```python
from build123d import *

# Parameters (mm, degrees)
EXTRUDE_1_DEPTH              = 7
CUT_EXTRUDE_1_DEPTH          = 4
HOLE_WIZARD_M3_1_D           = 3.4
HOLE_WIZARD_M3_1_DEPTH       = 7.5
HOLE_WIZARD_M3_1_CSINK_D     = 6.72
HOLE_WIZARD_M3_1_CSINK_ANGLE = 90
HOLE_WIZARD_M3_1_TIP         = 1.021463052
HOLE_WIZARD_1_D              = 4.15
CUT_EXTRUDE_2_DEPTH          = 4
CHAMFER_1_SIZE               = 0.5


with BuildPart() as part:
    # 草图1 → 凸台-拉伸1 (new body)
    with BuildSketch(Plane(origin=(0, 0, 0), x_dir=(1, 0, 0), z_dir=(0, 1, 0))):
        with BuildLine():
            Line((-4.25, 5), (4.25, 5))
            ThreePointArc((4.25, 5), (9.25, 0), (4.25, -5))
            Line((4.25, -5), (-4.25, -5))
            ThreePointArc((-4.25, -5), (-9.25, 0), (-4.25, 5))
        make_face()
    extrude(amount=EXTRUDE_1_DEPTH)

    # 草图2 → 切除-拉伸1 (cut)
    with BuildSketch(Plane(origin=(0, 7, 0), x_dir=(1, 0, 0), z_dir=(0, 1, 0))):
        with BuildLine():
            Line((-2.75, 2), (-5.75, 2))
            ThreePointArc((-5.75, 2), (-6.75, 0), (-5.75, -2))
            Line((-5.75, -2), (-2.75, -2))
            ThreePointArc((-2.75, -2), (-2.013932023, -1.118033989), (-1.75, 0))
            ThreePointArc((-1.75, 0), (-2.013932023, 1.118033989), (-2.75, 2))
        make_face()
    extrude(amount=-CUT_EXTRUDE_1_DEPTH, mode=Mode.SUBTRACT)

    # M3 六角凹锥坑螺钉的锥形沉头孔1
    with Locations(Plane(origin=(0, 0, 0), x_dir=(-1, 0, 0), z_dir=(0, -1, 0))):
        with Locations((4.25, 0)):
            CounterSinkHole(HOLE_WIZARD_M3_1_D / 2, HOLE_WIZARD_M3_1_CSINK_D / 2, depth=HOLE_WIZARD_M3_1_DEPTH, counter_sink_angle=HOLE_WIZARD_M3_1_CSINK_ANGLE)
            with Locations((0, 0, -(HOLE_WIZARD_M3_1_DEPTH + HOLE_WIZARD_M3_1_TIP / 2))):  # 118° drill point
                Cone(0, HOLE_WIZARD_M3_1_D / 2, HOLE_WIZARD_M3_1_TIP, mode=Mode.SUBTRACT)

    # 孔1 (through all)
    with Locations(Plane(origin=(0, 7, 0), x_dir=(1, 0, 0), z_dir=(0, 1, 0))):
        with Locations((5, -0.436816998)):
            Hole(HOLE_WIZARD_1_D / 2)

    # 草图12 → 切除-拉伸2 (cut)
    with BuildSketch(Plane(origin=(0, 7, 0), x_dir=(1, 0, 0), z_dir=(0, 1, 0))):
        Polygon((8.348631561, -0.436816998), (6.674315781, 2.463183002), (3.325684219, 2.463183002), (1.651368439, -0.436816998), (3.325684219, -3.336816998), (6.674315781, -3.336816998), align=None)
    extrude(amount=-CUT_EXTRUDE_2_DEPTH, mode=Mode.SUBTRACT)

    # 倒角1
    chamfer_1_edges = [part.edges().sort_by_distance(p)[0] for p in [
        (9.25, 7, 0),
        (0, 7, -5),
        (-9.25, 7, 0),
        (0, 0, -5),
        (9.25, 0, 0),
        (0, 0, 5),
        (-9.25, 0, 0),
        (0, 7, 5),
    ]]
    chamfer(chamfer_1_edges, length=CHAMFER_1_SIZE)


solid = part.part
```
Source: CAD feature listing. Evaluate the final solid. Frame: model axes, mm. A direction names the side the tool comes from. Round coordinates to 2 decimals unless told otherwise and drop trailing zeros. Loops run counter-clockwise (first coordinate to the right, second up) from the corner with the lowest first, then second, coordinate; pieces in that order, holes last. Notation, with made-up numbers: M 20.25,53 L 26.25,53 A19 cw 26.25,57 Z; hole C -24.75,78.5 d9. An arc over 180 degrees is marked long. Use a Markdown table: item, result. Add a question column.
1. Contact query for flat-ended pins moving along their axis: P1, Ø5, axis at x = 4.5, z = -2, coming from the +Y side; P2, Ø1.2, axis at x = -3, z = 0.5, coming from the +Y side; P3, Ø4, axis at x = -4.25, z = 0, coming from the -Y side; P4, Ø1, axis at x = 4, z = 0.5, coming from the +Y side. Output: stop coordinate, or through.
2. Reachability of faces 4 (the flat face through (5, 5, -2.463)), 5 (the cylindrical face through (-9.25, 3.46, 0.11)) from +Z, -Z, +X, -X, +Y, -Y: full face, straight path, thin tool, end or side. Return the list, or none.
3. Section query D-D on z = -1. Give the number of separate pieces and of enclosed holes in the cut face, then the cut area to 3 significant figures.
4. Mould query, pull axis X, two halves, no side actions, for faces 1 (the cylindrical face through (9.25, 3.46, -0.11)), 2 (the flat face through (5, 5, 3.337)), 3 (the conical face through (-8.884, 6.865, 0.102)). Classes: pulls with the +X half, pulls with the -X half, needs draft (parallel to the pull), parting line crosses it, or undercut.
5. Section query A-A on y = 5.75. Return the cut outline in (x, z), then the cut area to 3 significant figures.
6. Section query C-C on y = 2. Return the cut outline in (x, z) (3 decimals), then the cut area to 3 significant figures.
7. Line query: line 1 (X direction, y = 2.75, z = 1.25); line 2 (X direction, y = 4.5, z = -0.25); line 3 (Z direction, x = -3.25, y = 4.25). Output: solid intervals per line, ascending.
8. Section query B-B on x = 4. Return the cut outline in (y, z).
Reported:
| question | item | result |
|---|---|---|
| 1 | P1 | stops at y = 7 |
| 1 | P2 | stops at y = 3 |
| 1 | P3 | stops at y = 1.36 |
| 1 | P4 | passes through |
| 2 | face 4 | +Y |
| 2 | face 5 | -X, +Y, -Y |
| 3 | separate pieces | 3 |
| 3 | enclosed holes | 0 |
| 3 | area | 68.7 mm² |
| 4 | face 1 | pulls with the +X half |
| 4 | face 2 | undercut |
| 4 | face 3 | pulls with the -X half |
| 5 | outline | M -4.25,-5 L 4.25,-5 A5 ccw 4.25,5 L -4.25,5 A5 ccw Z; hole M -5.75,-2 L -2.75,-2 A2.5 ccw -2.75,2 L -5.75,2 A2.5 ccw Z; hole M 1.65,0.44 L 3.33,-2.46 L 6.67,-2.46 L 8.35,0.44 L 6.67,3.34 L 3.33,3.34 Z |
| 5 | area | 117 mm² |
| 6 | outline | M -4.25,-5 L 4.25,-5 A5 ccw 4.25,5 L -4.25,5 A5 ccw Z; hole C -4.25,0 d3.4; hole C 5,0.437 d4.15 |
| 6 | area | 141 mm² |
| 7 | line 1 | x = -9.09 to -5.4, -3.1 to 3.09, 6.91 to 9.09 |
| 7 | line 2 | x = -9.24 to -6.74, -1.76 to 2.05, 7.95 to 9.24 |
| 7 | line 3 | z = -5 to -2, 2 to 5 |
| 8 | outline | M 0,-4.5 L 0.5,-5 L 6.5,-5 L 7,-4.5 L 7,-2.46 L 3,-2.46 L 3,-1.38 L 0,-1.38 Z; M 0,2.25 L 3,2.25 L 3,3.34 L 7,3.34 L 7,4.5 L 6.5,5 L 0.5,5 L 0,4.5 Z |
